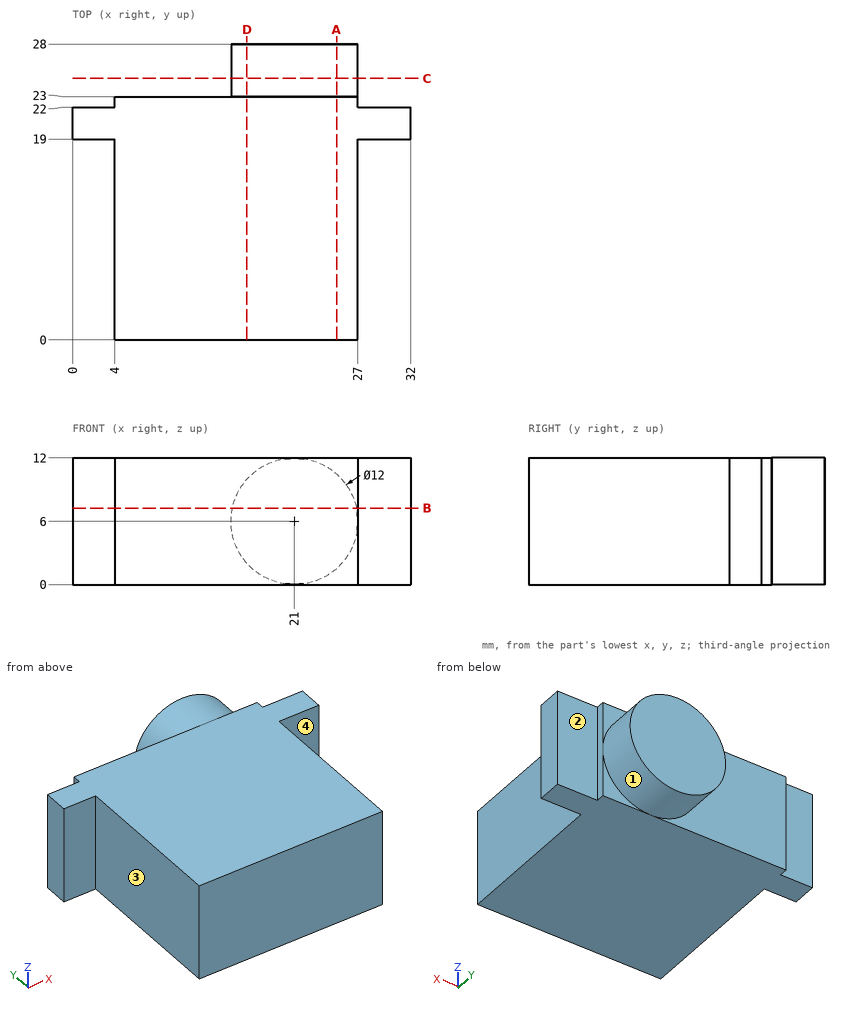
Study the drawing (mm; zero at the part's minimum x, y, z) and answer. A direction names the side the tool comes from. Coordinates: 2 decimals unless noted, no trailing zeros. Loops run counter-clockwise (first coordinate to the right, second up) from the corner with the lowest first, then second, coordinate; pieces in that order, holes last. Notation, with made-up numbers: M 54.25,76 L 62.25,76 A14 cw 62.25,101 Z; hole C 32,52.5 d7. An arc over 180 degrees is marked long. Answer in a Markdown table with one row per item.
1) Given pin 1 (1.2 mm diameter, centred on x = 1.5, z = 5, fed in from -Y); pin 2 (1.5 mm diameter, centred on x = 28, y = 25, fed in from +Z); pin 3 (6 mm diameter, centred on y = 11, z = 4, fed in from +X); pin 4 (2 mm diameter, centred on x = 1.5, z = 4, fed in from +Y), each flat-ended and moving along its own axis, determine where each tip first touches the part or whether it passes through.
Answers below:
| item | result |
|---|---|
| pin 1 | y = 19 |
| pin 2 | through |
| pin 3 | x = 27 |
| pin 4 | y = 22 |
2) Which of the six approach directions +Z, -Z, +X, -X, +Y, -Y give full straight-line access (tool end or side, diameter ignored) to the marked faces 1, 2, 3 and 4?
Answers below:
| item | result |
|---|---|
| face 1 | +Y |
| face 2 | +Z, -Z, +X, +Y |
| face 3 | +Z, -Z, -X, -Y |
| face 4 | +Z, -Z, +X, -Y |
3) Find the intervals of material crossed by probe 1 along Y at (x, z) = (27.5, 11.75); probe 2 along X at (y, z) = (13.5, 8.75); probe 3 along Y at (x, z) = (9.5, 2), in increasing order.
Answers below:
| item | result |
|---|---|
| probe 1 | 19 to 22 |
| probe 2 | 4 to 27 |
| probe 3 | 0 to 23 |
4) Find section D-D (x = 16.5). Determine the outline of the cut face in (y, z), then the cut area to 3 significant figures.
Answers below:
| item | result |
|---|---|
| outline | M 0,0 L 23,0 L 23,2.03 L 28,2.03 L 28,9.97 L 23,9.97 L 23,12 L 0,12 Z |
| area | 316 mm^2 |
5) Find section C-C (y = 24.75). Determine the outline of the cut face in (x, z), then the cut area to 3 significant figures.
Answers below:
| item | result |
|---|---|
| outline | C 21,6 d12 |
| area | 113 mm^2 |
6) Find section A-A (x = 25). Determine the outline of the cut face in (y, z).
Answers below:
| item | result |
|---|---|
| outline | M 0,0 L 23,0 L 23,1.53 L 28,1.53 L 28,10.47 L 23,10.47 L 23,12 L 0,12 Z |
7) Find section B-B (z = 7.25). Determine the outline of the cut face in (x, y), then the cut area to 3 significant figures.
Answers below:
| item | result |
|---|---|
| outline | M 0,19 L 4,19 L 4,0 L 27,0 L 27,19 L 32,19 L 32,22 L 27,22 L 27,23 L 26.87,23 L 26.87,28 L 15.13,28 L 15.13,23 L 4,23 L 4,22 L 0,22 Z |
| area | 615 mm^2 |
